The listing builds one solid part. Answer for the finished solid, in the listing's coordinates (mm). A direction names the side the tool comes from. Give positions to 0.01 mm unless a question says otherwise; leave off trailing zeros. Order: outer loops, then holes, each group sorted by start corner. A loop starts at its lowest first (then second) coordinate and runs counter-clockwise, first axis right, second up. Notation, with made-up numbers: (-17, -30.5) - (-10, -30.5) arc R35 ccw to (-10, 4.5) - close; hole circle Ø10 at (-32.75, 87.5). An arc over 180 degrees is marked (long way). Use a Markdown table: item, result. Add a question column.
1) For faces 5 (the face through (-2, 6, -10)), 6 (the face through (-9.615, 3.944, -0.668)), 7 (the face through (-3.25, 2.46, -10.42)), 8 (the face through (0, 2.5, 4)), determine the directions among +Z, -Z, +X, -X, +Y, -Y from which every point of the face is accessible in a straight line to the end or side of a thin tool.
2) Flat-ended cylindrical pins translate along their axes: pin 1 (4 mm diameter, centred on x = -5.5, z = -10.5, fed in from -Y); pin 2 (6 mm diameter, centred on x = -1, z = -16.5, fed in from -Y); pin 3 (1.8 mm diameter, centred on x = 6, z = -10.32, fed in from -Y). Find the tip coordinate at first contact, or state that the pin passes through.
3) Straight lines are drawn through the part: line 1 (Z direction, x = 1.75, y = 1.5); line 2 (Y direction, x = 1.5, z = 6.5); line 3 (Z direction, x = 1.25, y = 3.75). For each, find the intervals that lie inside material, in ascending order.
4) Find section D-D, the plane x = -11. Determine the outline of the cut face in (y, z).
5) Find section B-B, the plane y = 1. Determine the outline of the cut face in (x, z), plus the area to 3 significant figures.
6) The mould has two halves that part along Z. Classify faces 1 (the face through (0, 1, 8.66)), 2 (the face through (10.285, 1.232, 4.495)), 3 (the face through (12.38, 6.73, 7.2)), 4 (the face through (0, 5.5, 4)): released by +Z, released by -Z, zero draft, split by the parting line, or undercut.
7) Find section C-C, the plane y = 4. Determine the outline of the cut face in (x, z), plus the area to 3 significant figures.
8) Find section A-A, the plane x = -6. Determine the outline of the cut face in (y, z).
from build123d import *

# Parameters (mm, degrees)
SKETCH1_R           = 1.5
BOSS_EXTRUDE1_DEPTH = 8
SKETCH2_W           = 26.485934179
SKETCH2_H           = 3
CUT_EXTRUDE3_DEPTH  = 8.75
SKETCH3_R           = 8.5
SKETCH3_R_2         = 1.5
SKETCH3_R_3         = 1
BOSS_EXTRUDE2_DEPTH = 8
SKETCH4_R           = 2.75
CUT_EXTRUDE4_DEPTH  = 5
SKETCH5_R           = 3.5
CUT_EXTRUDE5_DEPTH  = 2
SKETCH3_3_R         = 1
CUT_EXTRUDE6_DEPTH  = 32


with BuildPart() as part:
    # Sketch1 → Boss-Extrude1 (new body)
    with BuildSketch(Plane(origin=(0, 0, 0), x_dir=(1, 0, 0), z_dir=(0, 1, 0))):
        with BuildLine():
            Line((-2.598076211, 12.820508076), (-12.401923789, -4.160254038))
            ThreePointArc((-12.401923789, -4.160254038), (-12.401923789, -7.160254038), (-9.803847577, -8.660254038))
            Line((-9.803847577, -8.660254038), (9.803847577, -8.660254038))
            ThreePointArc((9.803847577, -8.660254038), (12.401923789, -7.160254038), (12.401923789, -4.160254038))
            Line((12.401923789, -4.160254038), (2.598076211, 12.820508076))
            ThreePointArc((2.598076211, 12.820508076), (0, 14.320508076), (-2.598076211, 12.820508076))
        make_face()
        with Locations(Location((0, 10.320508076, 0), (0, 0, 270))):
            Circle(SKETCH1_R, mode=Mode.SUBTRACT)
        with Locations(Location((-8.82025404, -4.169491924, 0), (0, 0, 270))):
            Circle(SKETCH1_R, mode=Mode.SUBTRACT)
        with Locations(Location((8.82025404, -4.169491924, 0), (0, 0, 90))):
            Circle(SKETCH1_R, mode=Mode.SUBTRACT)
    extrude(amount=BOSS_EXTRUDE1_DEPTH)

    # Sketch2 → Cut-Extrude3 (cut)
    with BuildSketch(Plane.XY.offset(8.660254038)):
        with Locations((0.054095799, 4)):
            Rectangle(SKETCH2_W, SKETCH2_H)
    extrude(amount=-CUT_EXTRUDE3_DEPTH, mode=Mode.SUBTRACT)

    # Sketch3 → Boss-Extrude2 (add)
    with BuildSketch(Plane(origin=(0, 0, 0), x_dir=(-1, 0, 0), z_dir=(0, -1, 0))):
        with Locations((0, 10.320508076)):
            Circle(SKETCH3_R)
        with Locations(Location((0, 10.320508076, 0), (0, 0, 270))):
            Circle(SKETCH3_R_2, mode=Mode.SUBTRACT)
        with Locations(Location((-6, 10.320508076, 0), (0, 0, 90))):
            Circle(SKETCH3_R_3, mode=Mode.SUBTRACT)
        with Locations(Location((6, 10.320508076, 0), (0, 0, 90))):
            Circle(SKETCH3_R_3, mode=Mode.SUBTRACT)
        with Locations(Location((0, 16.320508076, 0), (0, 0, 90))):
            Circle(SKETCH3_R_3, mode=Mode.SUBTRACT)
        with Locations((0, 4.320508076)):
            Circle(SKETCH3_R_3, mode=Mode.SUBTRACT)
    extrude(amount=-BOSS_EXTRUDE2_DEPTH)

    # Sketch4 → Cut-Extrude4 (cut)
    with BuildSketch(Plane.XZ):
        with Locations((-6, -10.320508076)):
            Circle(SKETCH4_R)
        with Locations((6, -10.320508076)):
            Circle(SKETCH4_R)
        with Locations((0, -16.320508076)):
            Circle(SKETCH4_R)
        with Locations(Location((0, -4.320508076, 0), (0, 0, 90))):
            Circle(SKETCH4_R)
    extrude(amount=-CUT_EXTRUDE4_DEPTH, mode=Mode.SUBTRACT)

    # Sketch5 → Cut-Extrude5 (cut)
    with BuildSketch(Plane(origin=(0, 8, 0), x_dir=(1, 0, 0), z_dir=(0, 1, 0))):
        with Locations(Location((0, 10.320508076, 0), (0, 0, 270))):
            Circle(SKETCH5_R)
    extrude(amount=-CUT_EXTRUDE5_DEPTH, mode=Mode.SUBTRACT)

    # Sketch3<3> → Cut-Extrude6 (cut)
    with BuildSketch(Plane(origin=(0, 0, 0), x_dir=(-1, 0, 0), z_dir=(0, -1, 0))):
        with Locations(Location((0, 4.320508076, 0), (0, 0, 270))):
            Circle(SKETCH3_3_R)
    extrude(amount=-CUT_EXTRUDE6_DEPTH, mode=Mode.SUBTRACT)


solid = part.part
The answers:
| question | item | result |
|---|---|---|
| 1 | face 5 | +Y |
| 1 | face 6 | -X, +Y, -Y |
| 1 | face 7 | -Y |
| 1 | face 8 | +Z, +X, -X |
| 2 | pin 1 | y = 5 |
| 2 | pin 2 | y = 0 |
| 2 | pin 3 | through |
| 3 | line 1 | -18.64 to -18.44, -14.2 to -6.44, -2.2 to 8.66 |
| 3 | line 2 | 0 to 2.5, 5.5 to 8 |
| 3 | line 3 | -13.87 to -11.15, -9.49 to -6.77, -1.87 to -0.09 |
| 4 | outline | (0, 1.73) - (2.5, 1.73) - (2.5, 8.41) - (0, 8.41) - close; (5.5, 1.73) - (8, 1.73) - (8, 8.41) - (5.5, 8.41) - close |
| 5 | outline | (-12.4, 4.16) - (-6.9, -5.36) arc R8.5 ccw to (-8.39, -8.96) arc R2.75 cw (long way) to (-8.39, -11.68) arc R8.5 ccw to (-1.36, -18.71) arc R2.75 cw (long way) to (1.36, -18.71) arc R8.5 ccw to (8.39, -11.68) arc R2.75 cw (long way) to (8.39, -8.96) arc R8.5 ccw to (6.9, -5.36) - (12.4, 4.16) arc R3 ccw to (9.8, 8.66) - (-9.8, 8.66) arc R3 ccw to start; hole circle Ø3 at (-8.82, 4.17); hole circle Ø5.5 at (0, -4.32); hole circle Ø3 at (0, -10.32); hole circle Ø3 at (8.82, 4.17) |
| 5 | area | 373 mm2 |
| 6 | face 1 | released by +Z |
| 6 | face 2 | undercut |
| 6 | face 3 | split by the parting line |
| 6 | face 4 | zero draft |
| 7 | outline | (-9.95, -0.09) - (-6.9, -5.36) arc R8.5 ccw to (-8.39, -8.96) arc R2.75 cw (long way) to (-8.39, -11.68) arc R8.5 ccw to (-1.36, -18.71) arc R2.75 cw (long way) to (1.36, -18.71) arc R8.5 ccw to (8.39, -11.68) arc R2.75 cw (long way) to (8.39, -8.96) arc R8.5 ccw to (6.9, -5.36) - (9.95, -0.09) - close; hole circle Ø5.5 at (0, -4.32); hole circle Ø3 at (0, -10.32) |
| 7 | area | 181 mm2 |
| 8 | outline | (0, -16.34) - (8, -16.34) - (8, -11.32) - (5, -11.32) - (5, -13.07) - (0, -13.07) - close; (0, -7.57) - (5, -7.57) - (5, -9.32) - (8, -9.32) - (8, 8.66) - (5.5, 8.66) - (5.5, -0.09) - (2.5, -0.09) - (2.5, 8.66) - (0, 8.66) - close |
